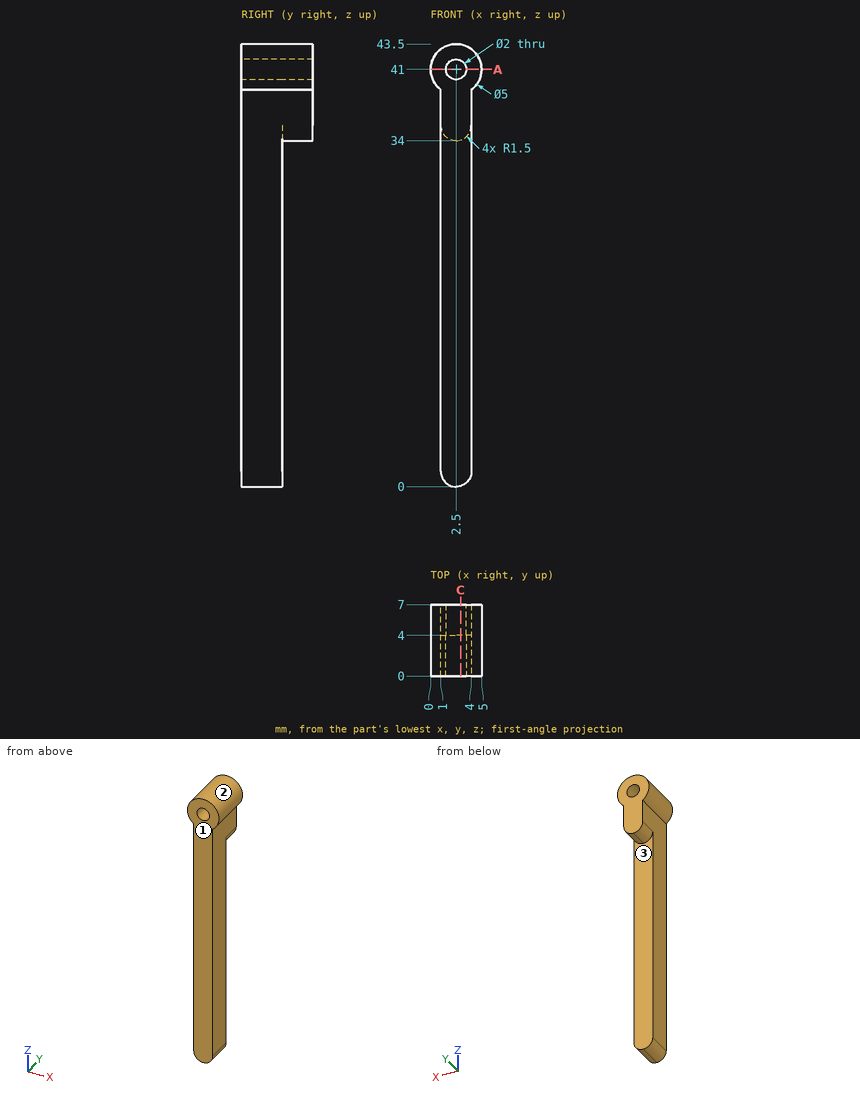
Geometry check sheet. Reference: drawing and pictorial views, mm from the part's lowest x, y, z. Coordinates: 2 decimals unless noted, no trailing zeros. Loops run counter-clockwise (first coordinate to the right, second up) from the corner with the lowest first, then second, coordinate; pieces in that order, holes last. Notation, with made-up numbers: (-25, -25.5) -> (10, -25.5) arc R36 cw to (10, 11.5) -> close; hole circle Ø4 at (27.25, -9). An arc over 180 degrees is marked (long way). Put each result on its own line as item: value.
1) Release check for a two-part mould opening along Y. For the marked faces 1, 2 and 3 record: released by +Y, released by -Y, zero draft, split by the parting line, or undercut.
Result set:
face 1: released by -Y
face 2: zero draft
face 3: released by +Y
2) Thickness scan on line 1 (X direction, y = 2, z = 41); line 2 (Z direction, x = 2.5, y = 5); line 3 (Z direction, x = 2.5, y = 2). Record the ranges inside material, lowest first.
Result set:
line 1: x = 0 to 1.5, 3.5 to 5
line 2: z = 34 to 40, 42 to 43.5
line 3: z = 0 to 40, 42 to 43.5
3) Cross-section at C-C on x = 2.95. Record the boundary of the cut face in (y, z), plus the area to 3 significant figures.
Result set:
outline: (0, 0.07) -> (4, 0.07) -> (4, 34.07) -> (7, 34.07) -> (7, 40.11) -> (0, 40.11) -> close; (0, 41.89) -> (7, 41.89) -> (7, 43.46) -> (0, 43.46) -> close
area: 189 mm^2
4) Gauge pin test, flat ends, axial feed: pin 1 Ø4 at (y, z) = (0.5, 20.5) entering from +X; pin 2 Ø3.5 at (y, z) = (2.5, 22) entering from -X; pin 3 Ø1.5 at (x, y) = (3.5, 4) entering from -Z. Record the tip position at first contact, or that the pin passes through.
Result set:
pin 1: stops at x = 4
pin 2: stops at x = 1
pin 3: stops at z = 0.02
5) Cross-section at A-A on z = 41. Record the boundary of the cut face in (x, y), plus the area to 3 significant figures.
Result set:
outline: (0, 0) -> (1.5, 0) -> (1.5, 7) -> (0, 7) -> close; (3.5, 0) -> (5, 0) -> (5, 7) -> (3.5, 7) -> close
area: 21.0 mm^2
